```python
from build123d import *

# Parameters (mm, degrees)
SKETCH1_R           = 1.7526
BOSS_EXTRUDE1_DEPTH = 3.175
CUT_EXTRUDE1_DEPTH  = 40.153784867
FILLET1_R           = 3.175


with BuildPart() as part:
    # Sketch1 → Boss-Extrude1 (new, symmetric)
    with BuildSketch(Plane.XY):
        with BuildLine():
            Line((-17.2212, 29.718), (-17.2212, -13.589))
            ThreePointArc((-17.2212, -13.589), (-16.29126403, -15.83406403), (-14.0462, -16.764))
            Line((-14.0462, -16.764), (21.5138, -16.764))
            ThreePointArc((21.5138, -16.764), (23.75886403, -15.83406403), (24.6888, -13.589))
            Line((24.6888, -13.589), (24.6888, -3.175))
            ThreePointArc((24.6888, -3.175), (23.75886403, -0.92993597), (21.5138, 0))
            Line((21.5138, 0), (3.175, 0))
            ThreePointArc((3.175, 0), (0.92993597, 0.92993597), (0, 3.175))
            Line((0, 3.175), (0, 29.718))
            Line((0, 29.718), (-17.2212, 29.718))
        make_face()
        with Locations((-5.0292, 26.67)):
            Circle(SKETCH1_R, mode=Mode.SUBTRACT)
        with Locations((-5.0292, -9.398)):
            Circle(SKETCH1_R, mode=Mode.SUBTRACT)
        with Locations((8.4328, -9.398)):
            Circle(SKETCH1_R, mode=Mode.SUBTRACT)
    extrude(amount=BOSS_EXTRUDE1_DEPTH, both=True)

    # Sketch2 → Cut-Extrude1 (cut, through all)
    with BuildSketch(Plane.XY.offset(3.175)):
        with BuildLine():
            Line((-5.0292, 22.225), (24.6888, 22.225))
            Line((24.6888, 22.225), (24.6888, 15.875))
            Line((24.6888, 15.875), (-5.0292, 15.875))
            ThreePointArc((-5.0292, 15.875), (-8.2042, 19.05), (-5.0292, 22.225))
        make_face()
    extrude(amount=-CUT_EXTRUDE1_DEPTH, mode=Mode.SUBTRACT)

    # Fillet1
    fillet1_edges = [part.edges().sort_by_distance(p)[0] for p in [
        (0, 15.875, 0),
        (0, 22.225, 0),
    ]]
    fillet(fillet1_edges, radius=FILLET1_R)


solid = part.part
```
CAD build for the part. Positions are in the model's coordinates, mm. A direction names the side the tool comes from. Round coordinates to 2 decimals unless told otherwise and drop trailing zeros. Write each loop counter-clockwise with the first axis right and the second up, starting at its lowest first coordinate (ties: lowest second). Pieces come first, ordered by that corner, then holes. Notation, with made-up numbers: (-2, 8.5) - (28, 8.5) arc R23 cw to (28, 20.5) - close; hole circle Ø8 at (-11.5, -18). An arc over 180 degrees is marked (long way). Return JSON: item names as keys, results as strings. Group by question number.
Item 1: 3-axis set-ups, long thin cutter, end or side, ignore diameter. For faces 4 (the face through (-16.316, -15.809, 0.044)), 5 (the face through (-0.955, 14.97, 0.044)), 6 (the face through (0, 28, 0)): which of +Z, -Z, +X, -X, +Y, -Y reach the whole face in a straight line?
Item 2: Mould opens along Y. For faces 1 (the face through (3, -16.764, 0)), 2 (the face through (0, 8, 0)), 3 (the face through (-6.42, 25.604, -0.044)) say: +Y half, -Y half, draft (parallel to the pull), parting line (faces both ways), or undercut.
Item 3: Band-saw the part on C-C on y = 19.05. List the corners of the cut face in (x, z) (3 decimals).
Item 4: Flat gauge pins, fed straight in: pin 1 Ø3 at (x, y) = (-5.03, 26.67) entering from -Z; pin 2 Ø2 at (y, z) = (27.5, 1.5) entering from +X. Where does each tip first touch, or does it go through?
Item 5: Band-saw the part on D-D on x = 17.5. List the corners of the cut face in (y, z) (3 decimals), plus the area to 3 significant figures.
Item 6: Probe probe 1 along Y at (x, z) = (6.5, 0); probe 2 along X at (y, z) = (3.5, -2.5); probe 3 along X at (y, z) = (19, -0.5). List the from-to ranges inside material, lowest first.
Item 7: Band-saw the part on A-A on y = 26.67. List the corners of the cut face in (x, z) (3 decimals).
Item 8: Band-saw the part on B-B on z = 0. List the corners of the cut face in (x, y) (3 decimals), plus the area to 3 significant figures.
Resolved:
{
 "1": {"face 4": "+Z, -Z, -X, -Y", "face 5": "+Z, -Z, +X", "face 6": "+Z, -Z, +X, +Y"},
 "2": {"face 1": "-Y half", "face 2": "draft", "face 3": "undercut"},
 "3": {"outline": "(-17.221, -3.175) - (-8.204, -3.175) - (-8.204, 3.175) - (-17.221, 3.175) - close"},
 "4": {"pin 1": "passes through", "pin 2": "stops at x = 0"},
 "5": {"outline": "(-16.764, -3.175) - (0, -3.175) - (0, 3.175) - (-16.764, 3.175) - close", "area": "106 mm²"},
 "6": {"probe 1": "y = -16.76 to 0", "probe 2": "x = -17.22 to 0", "probe 3": "x = -17.22 to -8.2"},
 "7": {"outline": "(-17.221, -3.175) - (-6.782, -3.175) - (-6.782, 3.175) - (-17.221, 3.175) - close; (-3.277, -3.175) - (0, -3.175) - (0, 3.175) - (-3.277, 3.175) - close"},
 "8": {"outline": "(-17.221, -13.589) arc R3.175 ccw to (-14.046, -16.764) - (21.514, -16.764) arc R3.175 ccw to (24.689, -13.589) - (24.689, -3.175) arc R3.175 ccw to (21.514, 0) - (3.175, 0) arc R3.175 cw to (0, 3.175) - (0, 12.7) arc R3.175 ccw to (-3.175, 15.875) - (-5.029, 15.875) arc R3.175 cw to (-5.029, 22.225) - (-3.175, 22.225) arc R3.175 ccw to (0, 25.4) - (0, 29.718) - (-17.221, 29.718) - close; hole circle Ø3.505 at (-5.029, -9.398); hole circle Ø3.505 at (-5.029, 26.67); hole circle Ø3.505 at (8.433, -9.398)", "area": "1,130 mm²"}
}
